For this review, take the finished solid that the model builds, in its own axes (mm). A direction names the side the tool comes from. Give positions to 0.01 mm unless a question says otherwise; leave off trailing zeros. One line per item, written item: value. Start each with the question number.
from build123d import *

# Parameters (mm, degrees)
ESQUISSE1_W        = 290
ESQUISSE1_H        = 120
BOSS_EXTRU_1_DEPTH = 5
CONG_1_R           = 1
CONG_2_R           = 1
ESQUISSE2_R        = 1.5
BOSS_EXTRU_2_DEPTH = 5
CONG_3_R           = 0.5
CHANFREIN1_SIZE    = 0.5


with BuildPart() as part:
    # Esquisse1 → Boss.-Extru.1 (new body)
    with BuildSketch(Plane.XY):
        Rectangle(ESQUISSE1_W, ESQUISSE1_H)
        with BuildLine():
            Line((-135, 2.5), (135, 2.5))
            ThreePointArc((135, 2.5), (137.5, 0), (135, -2.5))
            Line((135, -2.5), (-135, -2.5))
            ThreePointArc((-135, -2.5), (-137.5, 0), (-135, 2.5))
        make_face(mode=Mode.SUBTRACT)
        with BuildLine():
            Line((-135, 7.5), (135, 7.5))
            ThreePointArc((135, 7.5), (137.5, 10), (135, 12.5))
            Line((135, 12.5), (-135, 12.5))
            ThreePointArc((-135, 12.5), (-137.5, 10), (-135, 7.5))
        make_face(mode=Mode.SUBTRACT)
        with BuildLine():
            Line((-135, 17.5), (135, 17.5))
            ThreePointArc((135, 17.5), (137.5, 20), (135, 22.5))
            Line((135, 22.5), (-135, 22.5))
            ThreePointArc((-135, 22.5), (-137.5, 20), (-135, 17.5))
        make_face(mode=Mode.SUBTRACT)
        with BuildLine():
            Line((-135, 27.5), (135, 27.5))
            ThreePointArc((135, 27.5), (137.5, 30), (135, 32.5))
            Line((135, 32.5), (-135, 32.5))
            ThreePointArc((-135, 32.5), (-137.5, 30), (-135, 27.5))
        make_face(mode=Mode.SUBTRACT)
        with BuildLine():
            Line((-135, 37.5), (135, 37.5))
            ThreePointArc((135, 37.5), (137.5, 40), (135, 42.5))
            Line((135, 42.5), (-135, 42.5))
            ThreePointArc((-135, 42.5), (-137.5, 40), (-135, 37.5))
        make_face(mode=Mode.SUBTRACT)
        with BuildLine():
            Line((-135, 47.5), (135, 47.5))
            ThreePointArc((135, 47.5), (137.5, 50), (135, 52.5))
            Line((135, 52.5), (-135, 52.5))
            ThreePointArc((-135, 52.5), (-137.5, 50), (-135, 47.5))
        make_face(mode=Mode.SUBTRACT)
        with BuildLine():
            Line((-135, -12.5), (135, -12.5))
            ThreePointArc((135, -12.5), (137.5, -10), (135, -7.5))
            Line((135, -7.5), (-135, -7.5))
            ThreePointArc((-135, -7.5), (-137.5, -10), (-135, -12.5))
        make_face(mode=Mode.SUBTRACT)
        with BuildLine():
            Line((-135, -22.5), (135, -22.5))
            ThreePointArc((135, -22.5), (137.5, -20), (135, -17.5))
            Line((135, -17.5), (-135, -17.5))
            ThreePointArc((-135, -17.5), (-137.5, -20), (-135, -22.5))
        make_face(mode=Mode.SUBTRACT)
        with BuildLine():
            Line((-135, -32.5), (135, -32.5))
            ThreePointArc((135, -32.5), (137.5, -30), (135, -27.5))
            Line((135, -27.5), (-135, -27.5))
            ThreePointArc((-135, -27.5), (-137.5, -30), (-135, -32.5))
        make_face(mode=Mode.SUBTRACT)
        with BuildLine():
            Line((-135, -42.5), (135, -42.5))
            ThreePointArc((135, -42.5), (137.5, -40), (135, -37.5))
            Line((135, -37.5), (-135, -37.5))
            ThreePointArc((-135, -37.5), (-137.5, -40), (-135, -42.5))
        make_face(mode=Mode.SUBTRACT)
        with BuildLine():
            Line((-135, -52.5), (135, -52.5))
            ThreePointArc((135, -52.5), (137.5, -50), (135, -47.5))
            Line((135, -47.5), (-135, -47.5))
            ThreePointArc((-135, -47.5), (-137.5, -50), (-135, -52.5))
        make_face(mode=Mode.SUBTRACT)
    extrude(amount=BOSS_EXTRU_1_DEPTH)

    # Congé1
    cong_1_edges = [part.edges().sort_by_distance(p)[0] for p in [
        (0, -60, 5),
        (0, -60, 0),
    ]]
    fillet(cong_1_edges, radius=CONG_1_R)

    # Congé2
    cong_2_edges = [part.edges().sort_by_distance(p)[0] for p in [
        (0, 60, 0),
        (0, 60, 5),
    ]]
    fillet(cong_2_edges, radius=CONG_2_R)

    # Esquisse2 → Boss.-Extru.2 (add)
    # profile 1 of 2: a face of its own
    with BuildSketch(Plane(origin=(145, 0, 0), x_dir=(0, 0, -1), z_dir=(1, 0, 0))):
        with BuildLine():
            Line((-5, 20), (-15, 20))
            ThreePointArc((-15, 20), (-19.202041029, 30), (-15, 40))
            Line((-15, 40), (-5, 40))
            Line((-5, 40), (-5, 20))
        make_face()
        with Locations(Location((-10, 30, 0), (0, 0, 90))):
            Circle(ESQUISSE2_R, mode=Mode.SUBTRACT)
    # profile 2 of 2: a face of its own
    with BuildSketch(Plane(origin=(145, 0, 0), x_dir=(0, 0, -1), z_dir=(1, 0, 0))):
        with BuildLine():
            Line((-5, -20), (-5, -40))
            Line((-5, -40), (-15, -40))
            ThreePointArc((-15, -40), (-19.202041029, -30), (-15, -20))
            Line((-15, -20), (-5, -20))
        make_face()
        with Locations(Location((-10, -30, 0), (0, 0, 270))):
            Circle(ESQUISSE2_R, mode=Mode.SUBTRACT)
    boss_extru_2 = extrude(amount=-BOSS_EXTRU_2_DEPTH)

    # Symétrie1: Boss.-Extru.2 across plane
    add(boss_extru_2.mirror(Plane(origin=(0, 0, 0), x_dir=(0, 0, 1), z_dir=(1, 0, 0))))

    # Congé3
    cong_3_edges = [part.edges().sort_by_distance(p)[0] for p in [
        (140, -30, 5),
        (142.5, -20, 5),
        (142.5, -40, 5),
    ]]
    fillet(cong_3_edges, radius=CONG_3_R)

    # Chanfrein1
    chanfrein1_edges = [part.edges().sort_by_distance(p)[0] for p in [
        (140, 28.5, 10),
        (140, -28.5, 10),
        (-140, 28.5, 10),
        (-140, -28.5, 10),
    ]]
    chamfer(chanfrein1_edges, length=CHANFREIN1_SIZE)


solid = part.part
Q1. For pin 1 Ø4 at (x, z) = (-142.5, 9.5) entering from -Y; pin 2 Ø5 at (x, y) = (90, 1.5) entering from +Z, all flat-tipped, find the tip position at first contact; note any pin that passes through.
Q2. Take a section at A-A (x = -114.5). State how many separate pieces and enclosed holes the cut face has, and give its area (3 significant figures).
Q3. Mouldability with a two-part tool opening along X and no side actions: class faces 3 (the flat face through (2, 42.5, 2)), 4 (the flat face through (-143, -40, 10)) as pulls with the +X half, pulls with the -X half, needs draft (parallel to the pull), parting line crosses it, or undercut.
Q4. For faces 1 (the flat face through (2, -7.5, 2)), 2 (the flat face through (143, 20, 10)), list the 3-axis set-ups (+Z, -Z, +X, -X, +Y, -Y) from which the entire face can be reached by the end or side of a thin tool; tool diameter is ignored.
Q5. For line 1 along Z through (x, y) = (-143.35, 30); line 2 along X through (y, z) = (39, 10.5); line 3 along Z through (x, y) = (24.5, -46.5), list the stretches that pass through material, from the lowest coordinate up.
Answers below:
1. pin 1: stops at y = -40
1. pin 2: stops at z = 5
2. separate pieces: 12
2. enclosed holes: 0
2. area: 324 mm²
3. face 3: undercut
3. face 4: needs draft
4. face 1: +Z, -Z
4. face 2: +Z, +X, -X
5. line 1: z = 0 to 8.5, 11.5 to 19.2
5. line 2: x = -145 to -140, 140 to 145
5. line 3: z = 0 to 5
